Check sheet for the modelled part. Datum: model origin and axes. Units: mm. Face numbers are marked on the shaded views. A direction names the side the tool comes from. Give positions to 0.01 mm unless a question says otherwise; leave off trailing zeros. Loops run counter-clockwise (first coordinate to the right, second up) from the corner with the lowest first, then second, coordinate; pieces in that order, holes last. Notation, with made-up numbers: (-12, 51.25) -> (43, 51.25) arc R20 cw to (43, 60.25) -> close; hole circle Ø2 at (56, -0.5). An arc over 180 degrees is marked (long way). Answer as CSV lines item,"result". Start each with the question number.
(1) Section check D-D on x = 853. Enter the section's corners in (y, z).
(2) Section check C-C on z = -276. Enter the section's corners in (x, y), plus the area to 3 significant figures.
(3) Material ranges on line 1 (Y direction, x = 988, z = -75); line 2 (Y direction, x = 926, z = -6); line 3 (X direction, y = -233, z = -438.5), recorded low to high. Write a range as from..to.
(4) Release check for a two-part mould opening along Y. For the marked faces 1, 2, 3 and 4 record: pulls with the +Y half, pulls with the -Y half, needs draft (parallel to the pull), parting line crosses it, or undercut.
(5) Access from +Z, -Z, +X, -X, +Y, -Y to the whole of each face (thin tool, end or side, straight path). Record for the marked faces 5, 6 and 7.
(6) Section check A-A on y = -226.5. Enter the section's corners in (x, z).
(7) Gauge pin test, flat ends, axial feed: pin 1 Ø4 at (y, z) = (-122.5, -258) entering from +X; pin 2 Ø16 at (y, z) = (-524, -7) entering from -X. Record the tip position at first contact, or that the pin passes through.
(8) Section check B-B on x = 108. Enter the section's corners in (y, z), plus the area to 3 significant figures.
from build123d import *

# Parameters (mm, degrees)
SKETCH1_W               = 1200
SKETCH1_H               = 500
BOSS_EXTRUDE1_DEPTH     = 40
SKETCH2_W               = 50
SKETCH2_H               = 500
BOSS_EXTRUDE2_DEPTH     = 750
SKETCH3_W               = 650
SKETCH3_H               = 50
BOSS_EXTRUDE3_DEPTH     = 225
SKETCH4_W               = 50
SKETCH4_H               = 500
BOSS_EXTRUDE4_DEPTH     = 750
SKETCH5_W               = 370
SKETCH5_H               = 50
BOSS_EXTRUDE5_DEPTH     = 500
SKETCH6_W               = 370
SKETCH6_H               = 650
BOSS_EXTRUDE6_DEPTH     = 50
SKETCH7_W               = 330
SKETCH7_H               = 203
SKETCH7_H_2             = 204
BOSS_EXTRUDE7_DEPTH     = 450
SKETCH13_W              = 370
SKETCH13_H              = 650
SKETCH13_W_2            = 330
SKETCH13_H_2            = 610
BOSS_EXTRUDE9_DEPTH     = 450
SKETCH13_3_W            = 370
SKETCH13_3_H            = 650
SKETCH13_3_W_2          = 330
SKETCH13_3_H_2          = 610
CUT_EXTRUDE1_DEPTH      = 20
SKETCH14_W              = 330
SKETCH14_H              = 2
CUT_EXTRUDE_THIN1_DEPTH = 450


with BuildPart() as part:
    # Sketch1 → Boss-Extrude1 (new body)
    with BuildSketch(Plane(origin=(0, 0, 0), x_dir=(1, 0, 0), z_dir=(0, 1, 0))):
        with Locations((600, 250)):
            Rectangle(SKETCH1_W, SKETCH1_H)
    extrude(amount=BOSS_EXTRUDE1_DEPTH)

    # Sketch2 → Boss-Extrude2 (add)
    with BuildSketch(Plane.XZ):
        with Locations((40, -250)):
            Rectangle(SKETCH2_W, SKETCH2_H)
        with Locations((1160, -250)):
            Rectangle(SKETCH2_W, SKETCH2_H)
    extrude(amount=BOSS_EXTRUDE2_DEPTH)

    # Sketch3 → Boss-Extrude3 (add, symmetric)
    with BuildSketch(Plane.XY):
        with Locations((390, -125)):
            Rectangle(SKETCH3_W, SKETCH3_H)
    extrude(amount=BOSS_EXTRUDE3_DEPTH, both=True)

    # Sketch4 → Boss-Extrude4 (add)
    with BuildSketch(Plane.XZ):
        with Locations((740, -250)):
            Rectangle(SKETCH4_W, SKETCH4_H)
    extrude(amount=BOSS_EXTRUDE4_DEPTH)

    # Sketch5 → Boss-Extrude5 (add)
    with BuildSketch(Plane.XY):
        with Locations((950, -25)):
            Rectangle(SKETCH5_W, SKETCH5_H)
        with Locations((950, -725)):
            Rectangle(SKETCH5_W, SKETCH5_H)
    extrude(amount=-BOSS_EXTRUDE5_DEPTH)

    # Sketch6 → Boss-Extrude6 (add)
    with BuildSketch(Plane(origin=(0, 0, -500), x_dir=(-1, 0, 0), z_dir=(0, 0, -1))):
        with Locations((-950, -375)):
            Rectangle(SKETCH6_W, SKETCH6_H)
    extrude(amount=-BOSS_EXTRUDE6_DEPTH)

    # Sketch7 → Boss-Extrude7 (add)
    with BuildSketch(Plane.XY):
        with Locations((950, -171.5)):
            Rectangle(SKETCH7_W, SKETCH7_H)
        with Locations((950, -375)):
            Rectangle(SKETCH7_W, SKETCH7_H_2)
        with Locations((950, -578.5)):
            Rectangle(SKETCH7_W, SKETCH7_H)
    extrude(amount=-BOSS_EXTRUDE7_DEPTH)

    # Sketch13 → Boss-Extrude9 (add)
    with BuildSketch(Plane.XY):
        with Locations((950, -375)):
            Rectangle(SKETCH13_W, SKETCH13_H)
        with Locations((950, -375)):
            Rectangle(SKETCH13_W_2, SKETCH13_H_2, mode=Mode.SUBTRACT)
    extrude(amount=-BOSS_EXTRUDE9_DEPTH)

    # Sketch13_3 → Cut-Extrude1 (cut)
    with BuildSketch(Plane.XY):
        with Locations((950, -375)):
            Rectangle(SKETCH13_3_W, SKETCH13_3_H)
        with Locations((950, -375)):
            Rectangle(SKETCH13_3_W_2, SKETCH13_3_H_2, mode=Mode.SUBTRACT)
    extrude(amount=-CUT_EXTRUDE1_DEPTH, mode=Mode.SUBTRACT)

    # Sketch14 → Cut-Extrude-Thin1 (cut)
    with BuildSketch(Plane.XY):
        with Locations((950, -272)):
            Rectangle(SKETCH14_W, SKETCH14_H)
        with Locations((950, -476)):
            Rectangle(SKETCH14_W, SKETCH14_H)
    extrude(amount=-CUT_EXTRUDE_THIN1_DEPTH, mode=Mode.SUBTRACT)


solid = part.part
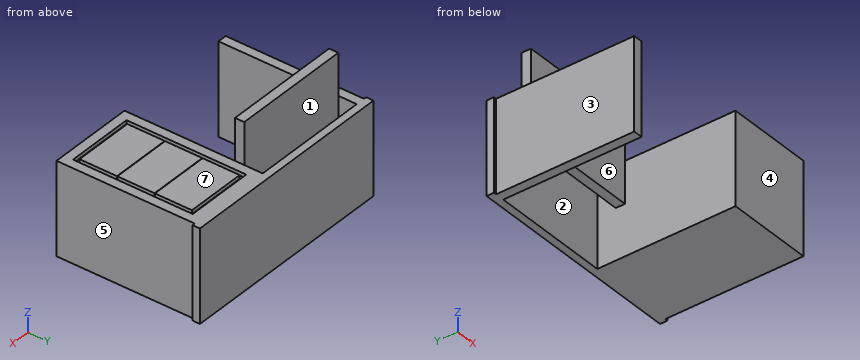
Working result:
1,outline,"(-750, -500) -> (40, -500) -> (40, 0) -> (-50, 0) -> (-50, -20) -> (-70, -20) -> (-70, 0) -> (-271, 0) -> (-271, -450) -> (-273, -450) -> (-273, 0) -> (-475, 0) -> (-475, -450) -> (-477, -450) -> (-477, 0) -> (-680, 0) -> (-680, -20) -> (-700, -20) -> (-700, 0) -> (-750, 0) -> close"
2,outline,"(0, 0) -> (15, 0) -> (15, -750) -> (65, -750) -> (65, 0) -> (715, 0) -> (715, -750) -> (1185, -750) -> (1185, 0) -> (1200, 0) -> (1200, 40) -> (0, 40) -> close; hole (785, -477) -> (1115, -477) -> (1115, -475) -> (785, -475) -> close; hole (785, -273) -> (1115, -273) -> (1115, -271) -> (785, -271) -> close"
2,area,"437,000 mm^2"
3,line 1,"y = -750..-477, -475..-273, -271..40"
3,line 2,"y = -750..-700, -680..-477, -475..-273, -271..-70, -50..40"
3,line 3,"x = 15..65, 715..1185"
4,face 1,"undercut"
4,face 2,"undercut"
4,face 3,"needs draft"
4,face 4,"pulls with the -Y half"
5,face 5,"+Z, -Z, +X, -Y"
5,face 6,"+Z, -Z, -Y"
5,face 7,"+Z, +X, +Y, -Y"
6,outline,"(15, -500) -> (65, -500) -> (65, 0) -> (15, 0) -> close; (715, -500) -> (1185, -500) -> (1185, 0) -> (1135, 0) -> (1135, -20) -> (1115, -20) -> (1115, 0) -> (785, 0) -> (785, -20) -> (765, -20) -> (765, 0) -> (715, 0) -> close"
7,pin 1,"stops at x = 1185"
7,pin 2,"stops at x = 15"
8,outline,"(-150, -225) -> (-100, -225) -> (-100, 225) -> (-150, 225) -> close; (0, -500) -> (40, -500) -> (40, 0) -> (0, 0) -> close"
8,area,"42,500 mm^2"
